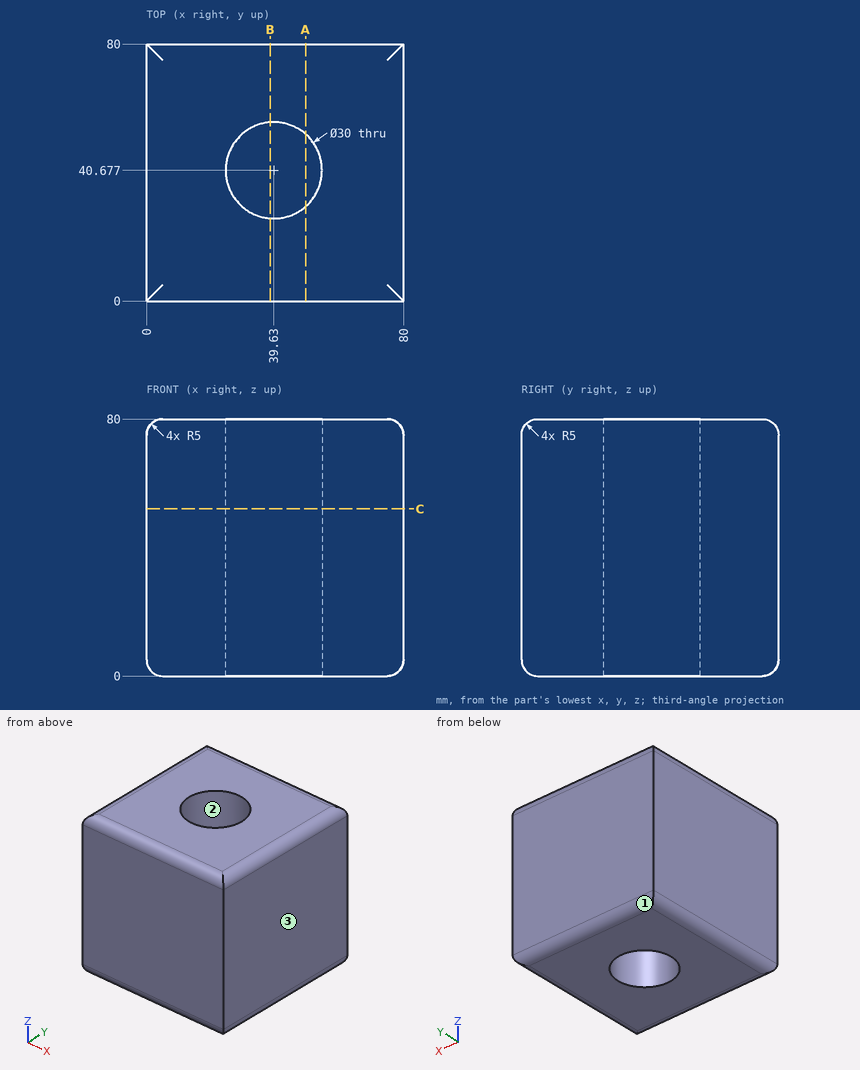
Study the drawing (mm; zero at the part's minimum x, y, z) and answer. Round coordinates to 2 decimals unless told otherwise and drop trailing zeros. Write each loop counter-clockwise with the first axis right and the second up, starting at its lowest first coordinate (ties: lowest second). Pieces come first, ordered by that corner, then holes.
1) A cutting plane is placed at C-C (z = 52). Give the vertices of the cut face in (x, y).
2) The mould has two halves that part along X. Classify the marked faces 1, 2 and 3: pulls with the +X half, pulls with the -X half, needs draft (parallel to the pull), parting line crosses it, or undercut.
3) A cutting plane is placed at A-A (x = 49.5). Give the vertices of the cut face in (y, z), plus the area to 3 significant figures.
4) Straight lines are drawn through the part: line 1 (X direction, y = 53, z = 44) (1 decimal); line 2 (Y direction, x = 45.5, z = 68); line 3 (X direction, y = 39, z = 37) (1 decimal). For each, find the intervals that lie inside material, in ascending order.
5) A cutting plane is placed at B-B (x = 38.5). Give the vertices of the cut face in (y, z) (1 decimal).
Completed:
1. outline: (0, 0) - (80, 0) - (80, 80) - (0, 80) - close; hole circle Ø30 at (39.63, 40.68)
2. face 1: needs draft
2. face 2: undercut
2. face 3: pulls with the +X half
3. outline: (0, 5) arc R5 ccw to (5, 0) - (29.38, 0) - (29.38, 80) - (5, 80) arc R5 ccw to (0, 75) - close; (51.97, 0) - (75, 0) arc R5 ccw to (80, 5) - (80, 75) arc R5 ccw to (75, 80) - (51.97, 80) - close
3. area: 4,570 mm2
4. line 1: x = 0 to 31.1, 48.2 to 80
4. line 2: y = 0 to 26.87, 54.48 to 80
4. line 3: x = 0 to 24.7, 54.5 to 80
5. outline: (0, 5) arc R5 ccw to (5, 0) - (25.7, 0) - (25.7, 80) - (5, 80) arc R5 ccw to (0, 75) - close; (55.6, 0) - (75, 0) arc R5 ccw to (80, 5) - (80, 75) arc R5 ccw to (75, 80) - (55.6, 80) - close
